from build123d import *

# Parameters (mm, degrees)
SKETCH_1_W      = 1610
SKETCH_1_H      = 805
SKETCH_1_W_2    = 1600
SKETCH_1_H_2    = 795
EXTRUDE_1_DEPTH = 50
SKETCH_1_7_W    = 1600
SKETCH_1_7_H    = 795
SKETCH_1_7_W_2  = 1510
SKETCH_1_7_H_2  = 705
EXTRUDE_2_DEPTH = 5


with BuildPart() as part:
    # Эскиз1 → Бобышка-Вытянуть1 (new body)
    with BuildSketch(Plane(origin=(0, 0, 0), x_dir=(1, 0, 0), z_dir=(0, 1, 0))):
        with Locations((693.181818182, 324.156044294)):
            Rectangle(SKETCH_1_W, SKETCH_1_H)
        with Locations((693.181818182, 324.156044294)):
            Rectangle(SKETCH_1_W_2, SKETCH_1_H_2, mode=Mode.SUBTRACT)
    extrude(amount=EXTRUDE_1_DEPTH)

    # Эскиз1<7> → Бобышка-Вытянуть2 (add)
    with BuildSketch(Plane(origin=(0, 0, 0), x_dir=(1, 0, 0), z_dir=(0, 1, 0))):
        with Locations((693.181818182, 324.156044294)):
            Rectangle(SKETCH_1_7_W, SKETCH_1_7_H)
        with Locations((693.181818182, 324.156044294)):
            Rectangle(SKETCH_1_7_W_2, SKETCH_1_7_H_2, mode=Mode.SUBTRACT)
    extrude(amount=EXTRUDE_2_DEPTH)


solid = part.part
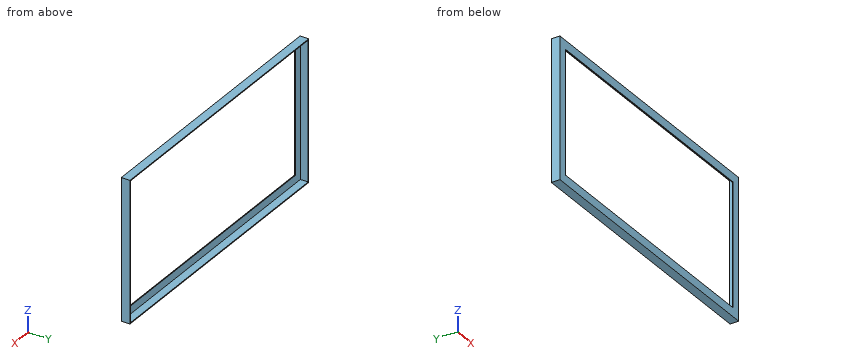
Design review of the part built by this model. Coordinates are the model's own, in mm. Round coordinates to 2 decimals unless told otherwise and drop trailing zeros. Loops run counter-clockwise (first coordinate to the right, second up) from the corner with the lowest first, then second, coordinate; pieces in that order, holes last. Notation, with made-up numbers: M 54,88 L 71,88 A14 ccw 71,112 Z; hole C 66.25,37 d6. An arc over 180 degrees is marked long. Answer as a JSON object with one key per item and string values.
Item 1: We need section C-C on y = 12.5. Give the boundary of the cut face in (x, z), and give its area (4 significant figures).
Answer sheet:
{"outline": "M -111.82,-726.66 L 1498.18,-726.66 L 1498.18,78.34 L -111.82,78.34 Z; hole M -106.82,-721.66 L 1493.18,-721.66 L 1493.18,73.34 L -106.82,73.34 Z", "area": "24,050 mm^2"}
Item 2: We need section B-B on x = 91.5. Give the boundary of the cut face in (y, z), and give its area (3 significant figures).
Answer sheet:
{"outline": "M 0,-726.66 L 50,-726.66 L 50,-721.66 L 5,-721.66 L 5,-676.66 L 0,-676.66 Z; M 0,28.34 L 5,28.34 L 5,73.34 L 50,73.34 L 50,78.34 L 0,78.34 Z", "area": "950 mm^2"}
Item 3: We need section A-A on z = -88.5. Give the boundary of the cut face in (x, y), and give its area (3 significant figures).
Answer sheet:
{"outline": "M -111.82,0 L -61.82,0 L -61.82,5 L -106.82,5 L -106.82,50 L -111.82,50 Z; M 1448.18,0 L 1498.18,0 L 1498.18,50 L 1493.18,50 L 1493.18,5 L 1448.18,5 Z", "area": "950 mm^2"}
Item 4: Wall thickness on L1, parallel to X at y = 4, z = -396; L2, parallel to Z at x = 958, y = 6.5; L3, parallel to X at y = 48, z = -588: over which ranges is each line inside the solid? List them lowest first. Write a range as from..to.
Answer sheet:
{"L1": "x = -111.82..-61.82, 1448.18..1498.18", "L2": "z = -726.66..-721.66, 73.34..78.34", "L3": "x = -111.82..-106.82, 1493.18..1498.18"}
